Autodesk Inventor part; units mm, degrees
ref_plane "YZ Plane" through (0, 0, 0) normal (1, 0, 0) x (0, 1, 0)
ref_plane "XZ Plane" through (0, 0, 0) normal (0, 1, 0) x (-1, 0, 0)
ref_plane "XY Plane" through (0, 0, 0) normal (0, 0, 1) x (1, 0, 0)
sketch "スケッチ1" plane through (0, 0, 0) normal (0, 1, 0) x (-1, 0, 0)
  circle A0 centre (0, 0) radius 4
  circle A1 centre (0, 0) radius 8
  circle A2 centre (0, 0) radius 6 construction
  circle A3 centre (0, -6) radius 1.1
  circle A4 centre (4.2426, -4.2426) radius 1.1
  circle A5 centre (6, 0) radius 1.1
  circle A6 centre (4.2426, 4.2426) radius 1.1
  circle A7 centre (0, 6) radius 1.1
  circle A8 centre (-4.2426, 4.2426) radius 1.1
  circle A9 centre (-6, 0) radius 1.1
  circle A10 centre (-4.2426, -4.2426) radius 1.1
  line L0 (26.25, -15) -> (-26.25, -15)
  line L1 (-26.25, -15) -> (-26.25, 30)
  line L2 (-26.25, 30) -> (26.25, 30)
  line L3 (26.25, 30) -> (26.25, -15)
  line L4 (24.25, 11.5) -> (21.25, 11.5)
  line L5 (21.25, 11.5) -> (21.25, 21.5)
  line L6 (21.25, 21.5) -> (24.25, 21.5)
  line L7 (24.25, 21.5) -> (24.25, 11.5)
  circle A11 centre (24.25, 12.6) radius 1.1
  circle A12 centre (21.25, 12.6) radius 1.1
  line L8 (0, 0) -> (0, -15) construction
  circle A13 centre (24.25, 20.4) radius 1.1
  circle A14 centre (21.25, 20.4) radius 1.1
  line L9 (-24.25, 11.5) -> (-21.25, 11.5)
  line L10 (-21.25, 11.5) -> (-21.25, 21.5)
  line L11 (-21.25, 21.5) -> (-24.25, 21.5)
  line L12 (-24.25, 21.5) -> (-24.25, 11.5)
  circle A15 centre (-24.25, 12.6) radius 1.1
  circle A16 centre (-21.25, 12.6) radius 1.1
  circle A17 centre (-24.25, 20.4) radius 1.1
  circle A18 centre (-21.25, 20.4) radius 1.1
  circle A19 centre (22.75, 6.5) radius 1.1
  circle A20 centre (22.75, 26.5) radius 1.1
  circle A21 centre (-22.75, 6.5) radius 1.1
  circle A22 centre (-22.75, 26.5) radius 1.1
  circle A23 centre (22.75, 26.5) radius 3.5 construction
  point P0 (21.25, 16.5)
  point P1 (-21.25, 16.5)
  point P2 (22.75, 11.5)
  point P3 (-21.25, 19.3)
  point P4 (-21.25, 13.7)
  point P5 (-24.25, 13.7)
  point P6 (-24.25, 19.3)
  point P7 (-24.25, 21.5)
  point P8 (-21.25, 21.5)
  point P9 (21.25, 19.3)
  point P10 (21.25, 21.5)
  point P11 (24.25, 21.5)
  point P12 (24.25, 19.3)
  point P13 (24.25, 13.7)
  point P14 (21.25, 13.7)
  point P15 (22.75, 21.5)
  dimension "d2" = 12
  dimension "d10" = 2.2
  dimension "d0" = 8
  dimension "d1" = 16
  dimension "d3" = 2.2
  dimension "d6" = 360
  dimension "d8" = 3
  dimension "d9" = 10
  dimension "d11" = 42.5
  dimension "d12" = 2.2
  dimension "d13" = 5
  dimension "d17" = 5
  dimension "d18" = 7
  dimension "d29" = 45
  dimension "d30" = 30
extrude "押し出し1" add sketch "スケッチ1" along normal blind 1.5 contours A1 | L0 L1 L2 L3
sketch "スケッチ2" plane through (0, 0, 0) normal (0, -1, 0) x (1, 0, 0)
  circle A0 centre (-22.75, -5.5) radius 1.1
  circle A1 centre (-22.75, 6.5) radius 1.1
  point P0 (0, 0)
  dimension "d19" = 2.2
  dimension "d20" = 12
extrude "押し出し2" cut sketch "スケッチ2" against normal through all contours A0
fillet "フィレット1" radius 2 4 edges at (-26.25, 0.75, -15) (26.25, 0.75, -15) (26.25, 0.75, 30) (-26.25, 0.75, 30)
sketch "スケッチ4" plane through (0, 0, 0) normal (0, -1, 0) x (1, 0, 0)
  circle A0 centre (0, 0) radius 8
  circle A1 centre (0, -6) radius 1.1
  circle A2 centre (0, -6) radius 2
  circle A3 centre (-22.75, -5.5) radius 1.1
  arc A4 (-24.25, 30) -> (-26.25, 28) centre (-24.25, 28) ccw
  line L0 (-26.25, -13) -> (-26.25, 28)
  arc A5 (-26.25, -13) -> (-24.25, -15) centre (-24.25, -13) ccw
  line L1 (24.25, -15) -> (-24.25, -15)
  arc A6 (24.25, -15) -> (26.25, -13) centre (24.25, -13) ccw
  line L2 (26.25, 28) -> (26.25, -13)
  arc A7 (26.25, 28) -> (24.25, 30) centre (24.25, 28) ccw
  line L3 (-24.25, 30) -> (24.25, 30)
  circle A8 centre (22.75, 26.5) radius 1.1
  circle A9 centre (-22.75, 26.5) radius 1.1
  circle A10 centre (-22.75, 6.5) radius 1.1
  line L4 (21.25, 19.3) -> (21.25, 13.7)
  arc A11 (21.25, 21.5) -> (21.25, 19.3) centre (21.25, 20.4) ccw
  line L5 (24.25, 21.5) -> (21.25, 21.5)
  arc A12 (24.25, 19.3) -> (24.25, 21.5) centre (24.25, 20.4) ccw
  line L6 (24.25, 13.7) -> (24.25, 19.3)
  arc A13 (24.25, 11.5) -> (24.25, 13.7) centre (24.25, 12.6) ccw
  line L7 (21.25, 11.5) -> (24.25, 11.5)
  arc A14 (21.25, 13.7) -> (21.25, 11.5) centre (21.25, 12.6) ccw
  arc A15 (-21.25, 19.3) -> (-21.25, 21.5) centre (-21.25, 20.4) ccw
  line L8 (-21.25, 13.7) -> (-21.25, 19.3)
  arc A16 (-21.25, 11.5) -> (-21.25, 13.7) centre (-21.25, 12.6) ccw
  line L9 (-24.25, 11.5) -> (-21.25, 11.5)
  arc A17 (-24.25, 13.7) -> (-24.25, 11.5) centre (-24.25, 12.6) ccw
  line L10 (-24.25, 19.3) -> (-24.25, 13.7)
  arc A18 (-24.25, 21.5) -> (-24.25, 19.3) centre (-24.25, 20.4) ccw
  line L11 (-21.25, 21.5) -> (-24.25, 21.5)
  circle A19 centre (6, 0) radius 1.1
  circle A20 centre (0, 6) radius 1.1
  circle A21 centre (-6, 0) radius 1.1
  circle A22 centre (0, -6) radius 1.1
  circle A23 centre (22.75, 6.5) radius 1.1
  circle A24 centre (4.2426, -4.2426) radius 1.1
  circle A25 centre (4.2426, 4.2426) radius 1.1
  circle A26 centre (-4.2426, 4.2426) radius 1.1
  circle A27 centre (-4.2426, -4.2426) radius 1.1
  circle A28 centre (0, 0) radius 4
  line L12 (-17.15, -5.9) -> (-17.15, 20.9)
  line L13 (-17.15, 20.9) -> (17.15, 20.9)
  line L14 (17.15, 20.9) -> (17.15, -5.9)
  line L15 (17.15, -5.9) -> (-17.15, -5.9)
  arc A29 (21.25, 13.7) -> (21.25, 11.5) centre (21.25, 12.6) ccw
  line L16 (0, 0) -> (17.15, 20.9) construction
  line L17 (0, 0) -> (0, 20.9) construction
  line L18 (19.4692, 18.997) -> (2.3192, -1.903)
  line L19 (2.3192, -1.903) -> (-2.3192, 1.903) construction
  line L20 (-2.3192, 1.903) -> (14.8308, 22.803)
  line L21 (14.8308, 22.803) -> (19.4692, 18.997) construction
  line L22 (19.4692, 18.997) -> (-2.3192, 1.903) construction
  line L23 (2.3192, -1.903) -> (14.8308, 22.803) construction
  line L24 (-19.4692, 18.997) -> (-2.3192, -1.903)
  line L25 (2.3192, 1.903) -> (-14.8308, 22.803)
  point P0 (20.15, 12.6)
  point P1 (8.575, 10.45)
  point P2 (-7.0236, 3.8301)
  point P3 (-17.15, 16.1707)
  point P4 (-5.4028, -5.9)
  point P5 (-13.2693, 20.9)
  point P6 (-2.3853, 7.6361)
  point P7 (2.3853, 7.6361)
  point P8 (13.2693, 20.9)
  point P9 (17.15, 16.1707)
  point P10 (7.0236, 3.8301)
  point P11 (5.4028, -5.9)
  dimension "d31" = 4
  dimension "d32" = 3
  dimension "d33" = 6
extrude "押し出し4" cut sketch "スケッチ4" against normal through all contours A0 L18 L14 L15 | A0 L25 L13 L20 | L15 L12 L24 A0
fillet "フィレット3" radius 2 12 edges at (13.2693, 0.75, 20.9) (17.15, 0.75, 16.1707) (17.15, 0.75, -5.9) (5.4028, 0.75, -5.9) (7.0236, 0.75, 3.8301) (2.3853, 0.75, 7.6361) (-2.3853, 0.75, 7.6361) (-13.2693, 0.75, 20.9) (-17.15, 0.75, 16.1707) (-7.0236, 0.75, 3.8301) (-5.4028, 0.75, -5.9) (-17.15, 0.75, -5.9)
properties part number "kosi_v3_1.5" material "アルミニウム 2014-T4"
Source: CAD feature listing. Evaluate the final solid. Frame: model axes, mm. A direction names the side the tool comes from. Round coordinates to 2 decimals unless told otherwise and drop trailing zeros. Loops run counter-clockwise (first coordinate to the right, second up) from the corner with the lowest first, then second, coordinate; pieces in that order, holes last. Notation, with made-up numbers: (-21.75, 68.25) - (32.25, 68.25) arc R14 ccw to (32.25, 74.25) - close; hole circle Ø8 at (-18, 65.25). An arc over 180 degrees is marked (long way). Write item = value, one per line. Start each with the question number.
(1) Section query C-C, the plane x = 16.5. Output: boundary loops of the cut face in (y, z), plus the area to 3 significant figures.
(2) Section query A-A, the plane z = 0. Output: boundary loops of the cut face in (x, y).
(3) Section query B-B, the plane x = -22.75. Output: boundary loops of the cut face in (y, z), plus the area to 3 significant figures.
(4) Pull-direction query (X, two-part tool) for faces 3 (the face through (-7.388, 0.76, 3.863)), 4 (the face through (-25.68, 0.76, 29.4)), 5 (the face through (0.4, 1.5, 7.8)); classes: +X half, -X half, draft (parallel to the pull), parting line (faces both ways), or undercut.
(5) Section query D-D, the plane z = 17. Output: boundary loops of the cut face in (x, y), plus the area to 3 significant figures.
(6) Set-up query: faces 1 (the face through (-26.25, 1, 8)), 2 (the face through (23, 1, 11.5)). Return all of +Z, -Z, +X, -X, +Y, -Y with unobstructed straight access to the full face (end or side cutting, diameter ignored); none if empty.
(7) Ray query, line 1 along Z through (x, y) = (0, 1.1); line 2 along Z through (x, y) = (22.5, 0.8); line 3 along Z through (x, y) = (-0.5, 1.25). Return the intervals inside material, ascending. Write a range as from..to.
Conclusion:
q1.outline = (0, -15) - (1.5, -15) - (1.5, -5.38) - (0, -5.38) - close; (0, 12.06) - (1.5, 12.06) - (1.5, 30) - (0, 30) - close
q1.area = 41.4 mm2
q2.outline = (-26.25, 0) - (-17.15, 0) - (-17.15, 1.5) - (-26.25, 1.5) - close; (-8, 0) - (-7.1, 0) - (-7.1, 1.5) - (-8, 1.5) - close; (-4.9, 0) - (-4, 0) - (-4, 1.5) - (-4.9, 1.5) - close; (4, 0) - (4.9, 0) - (4.9, 1.5) - (4, 1.5) - close; (7.1, 0) - (8, 0) - (8, 1.5) - (7.1, 1.5) - close; (17.15, 0) - (26.25, 0) - (26.25, 1.5) - (17.15, 1.5) - close
q3.outline = (0, -15) - (1.5, -15) - (1.5, -6.6) - (0, -6.6) - close; (0, -4.4) - (1.5, -4.4) - (1.5, 5.4) - (0, 5.4) - close; (0, 7.6) - (1.5, 7.6) - (1.5, 11.5) - (0, 11.5) - close; (0, 21.5) - (1.5, 21.5) - (1.5, 25.4) - (0, 25.4) - close; (0, 27.6) - (1.5, 27.6) - (1.5, 30) - (0, 30) - close
q3.area = 42.6 mm2
q4.face_3 = undercut
q4.face_4 = -X half
q4.face_5 = draft
q5.outline = (-26.25, 0) - (-24.25, 0) - (-24.25, 1.5) - (-26.25, 1.5) - close; (-21.25, 0) - (-10.07, 0) - (-10.07, 1.5) - (-21.25, 1.5) - close; (10.07, 0) - (21.25, 0) - (21.25, 1.5) - (10.07, 1.5) - close; (24.25, 0) - (26.25, 0) - (26.25, 1.5) - (24.25, 1.5) - close
q5.area = 39.5 mm2
q6.face_1 = +Z, -Z, -X, +Y, -Y
q6.face_2 = +Y, -Y
q7.line_1 = -15..-7.1, -4.9..-4, 4..4.9, 7.1..8, 20.9..30
q7.line_2 = -15..5.43, 7.57..11.5, 21.5..25.43, 27.57..30
q7.line_3 = -15..-6.98, -5.02..-3.97, 3.97..5.02, 6.98..7.98, 20.9..30
